from build123d import *

# Parameters (mm, degrees)
EXTRUDE_1_DEPTH = 15
SKETCH_2_R      = 1.15
EXTRUDE_2_DEPTH = 1.5
EXTRUDE_START   = 2.5
SKETCH_2_2_R    = 1.15
EXTRUDE_3_DEPTH = 1.5
FILLET_1_R      = 1
SKETCH_4_R      = 1
EXTRUDE_5_DEPTH = 4


with BuildPart() as part:
    # 草图1 → 凸台-拉伸1 (new body)
    with BuildSketch(Plane(origin=(0, 0, 0), x_dir=(1, 0, 0), z_dir=(0, 1, 0))):
        Polygon((-2, -2), (14.2, -2), (14.2, 12.2), (-2, 12.2), (-2, 5.6), (0, 5.6), (0, 10.2), (12.2, 10.2), (12.2, 0), (0, 0), (0, 4.6), (-2, 4.6), align=None)
    extrude(amount=EXTRUDE_1_DEPTH)

    # 草图2 → 凸台-拉伸2 (add)
    with BuildSketch(Plane.XY.offset(-5.6)):
        with BuildLine():
            Line((-4, 8.5), (-2, 8.5))
            Line((-2, 8.5), (-2, 4.5))
            Line((-2, 4.5), (-4, 4.5))
            ThreePointArc((-4, 4.5), (-6, 6.5), (-4, 8.5))
        make_face()
        with Locations((-4, 6.5)):
            Circle(SKETCH_2_R, mode=Mode.SUBTRACT)
    extrude(amount=-EXTRUDE_2_DEPTH)

    # 草图2<2> → 凸台-拉伸3 (add)
    with BuildSketch(Plane.XY.offset(-5.6).offset(EXTRUDE_START)):
        with BuildLine():
            Line((-4, 8.5), (-2, 8.5))
            Line((-2, 8.5), (-2, 4.5))
            Line((-2, 4.5), (-4, 4.5))
            ThreePointArc((-4, 4.5), (-6, 6.5), (-4, 8.5))
        make_face()
        with Locations((-4, 6.5)):
            Circle(SKETCH_2_2_R, mode=Mode.SUBTRACT)
    extrude(amount=-EXTRUDE_3_DEPTH)

    # 圆角1
    fillet_1_edges = [part.edges().sort_by_distance(p)[0] for p in [
        (0, 7.5, 0),
        (12.2, 7.5, 0),
        (12.2, 7.5, -10.2),
        (0, 7.5, -10.2),
    ]]
    fillet(fillet_1_edges, radius=FILLET_1_R)

    # 草图4 → 凸台-拉伸5 (add)
    # profile 1 of 3: a face of its own
    with BuildSketch(Plane(origin=(0, 12, 0), x_dir=(1, 0, 0), z_dir=(0, 1, 0))):
        with BuildLine():
            Line((5.1, -2), (5.1, -4.9))
            ThreePointArc((5.1, -4.9), (3.1, -6.9), (1.1, -4.9))
            Line((1.1, -4.9), (1.1, -2))
            Line((1.1, -2), (5.1, -2))
        make_face()
        with Locations(Location((3.1, -4.9, 0), (0, 0, 90))):
            Circle(SKETCH_4_R, mode=Mode.SUBTRACT)
    # profile 2 of 3: a face of its own
    with BuildSketch(Plane(origin=(0, 12, 0), x_dir=(1, 0, 0), z_dir=(0, 1, 0))):
        with BuildLine():
            Line((1.1, 15.1), (1.1, 12.2))
            Line((1.1, 12.2), (5.1, 12.2))
            Line((5.1, 12.2), (5.1, 15.1))
            ThreePointArc((5.1, 15.1), (3.1, 17.1), (1.1, 15.1))
        make_face()
        with Locations(Location((3.1, 15.1, 0), (0, 0, 270))):
            Circle(SKETCH_4_R, mode=Mode.SUBTRACT)
    # profile 3 of 3: a face of its own
    with BuildSketch(Plane(origin=(0, 12, 0), x_dir=(1, 0, 0), z_dir=(0, 1, 0))):
        with BuildLine():
            Line((17.1, 7.1), (14.2, 7.1))
            Line((14.2, 7.1), (14.2, 3.1))
            Line((14.2, 3.1), (17.1, 3.1))
            ThreePointArc((17.1, 3.1), (19.1, 5.1), (17.1, 7.1))
        make_face()
        with Locations(Location((17.1, 5.1, 0), (0, 0, 270))):
            Circle(SKETCH_4_R, mode=Mode.SUBTRACT)
    extrude(amount=-EXTRUDE_5_DEPTH)


solid = part.part
Check sheet for the modelled part. Datum: model origin and axes. Units: mm. A direction names the side the tool comes from. Round coordinates to 2 decimals unless told otherwise and drop trailing zeros. Loops run counter-clockwise (first coordinate to the right, second up) from the corner with the lowest first, then second, coordinate; pieces in that order, holes last. Notation, with made-up numbers: (-9, 68) - (16, 68) arc R11 cw to (16, 85) - close; hole circle Ø1 at (4, -6.5). An arc over 180 degrees is marked (long way). Answer as CSV lines item,"result". Start each with the question number.
Item 1: Scan lines: line 1 (Z direction, x = 2.25, y = 13.5); line 2 (X direction, y = 3, z = -4.5); line 3 (Y direction, x = -4, z = -4.05). Record each from-to range of solid material in increasing order. Write a range as [from, to].
Item 2: Section check C-C (y = 10). Count the separate pieces of the cut face and the enclosed holes in it, and give its area (3 significant figures).
Item 3: Section check D-D (x = 6.75). Record the boundary of the cut face in (y, z).
Item 4: Section check B-B (x = 1.5). Record the boundary of the cut face in (y, z).
Item 5: Release check for a two-part mould opening along X. For faces 1 (the cylindrical face through (3.1, 10, 6.9)), 2 (the flat face through (-3, 8.5, -4)), 3 (the flat face through (0, 7, -3)) record: +X half, -X half, draft (parallel to the pull), parting line (faces both ways), or undercut.
Item 6: Depth check by flat-ended pin: P1, Ø1.1, axis at y = 7, z = -7, coming from the +X side; P2, Ø5, axis at x = -2.5, y = 11, coming from the -Z side; P3, Ø3, axis at y = 9.5, z = -14.5, coming from the +X side. Enter the tip coordinate at first touch or a pass-through.
Item 7: Set-up check for faces 4 (the flat face through (5.1, 10, -14)), 5 (the flat face through (16, 8, -6)), 6 (the flat face through (1.1, 10, 3)), 7 (the flat face through (12.2, 7, -5)): record each of +Z, -Z, +X, -X, +Y, -Y from which the full face is reachable in a straight line by a thin tool's end or side.
Item 8: Section check A-A (z = -3.5). Record the boundary of the cut face in (x, y), and give its area (3 significant figures).
Report:
1,line 1,"z = [-12.2, -10.2], [0, 2]"
1,line 2,"x = [-2, 0], [12.2, 14.2]"
1,line 3,"y = [4.5, 5.35], [7.65, 8.5]"
2,separate pieces,"1"
2,enclosed holes,"3"
2,area,"149 mm2"
3,outline,"(0, -12.2) - (15, -12.2) - (15, -10.2) - (0, -10.2) - close; (0, 0) - (15, 0) - (15, 2) - (0, 2) - close"
4,outline,"(0, -12.2) - (8, -12.2) - (8, -16.3) - (12, -16.3) - (12, -12.2) - (15, -12.2) - (15, -10.2) - (0, -10.2) - close; (0, 0) - (15, 0) - (15, 2) - (12, 2) - (12, 6.1) - (8, 6.1) - (8, 2) - (0, 2) - close"
5,face 1,"parting line"
5,face 2,"draft"
5,face 3,"undercut"
6,P1,"stops at x = 14.2"
6,P2,"stops at z = -12.2"
6,P3,"stops at x = 5.1"
7,face 4,"-Z, +X, +Y, -Y"
7,face 5,"+Z, -Z, +X, -Y"
7,face 6,"+Z, -X, +Y, -Y"
7,face 7,"+Y, -Y"
8,outline,"(-4, 4.5) - (-2, 4.5) - (-2, 0) - (0, 0) - (0, 15) - (-2, 15) - (-2, 8.5) - (-4, 8.5) arc R2 ccw to start; (12.2, 0) - (14.2, 0) - (14.2, 8) - (18.3, 8) - (18.3, 12) - (14.2, 12) - (14.2, 15) - (12.2, 15) - close; hole circle Ø2.3 at (-4, 6.5)"
8,area,"86.5 mm2"
